Autodesk Inventor part; units mm, degrees
ref_plane "YZ Plane" through (0, 0, 0) normal (1, 0, 0) x (0, 1, 0)
ref_plane "XZ Plane" through (0, 0, 0) normal (0, 1, 0) x (-1, 0, 0)
ref_plane "XY Plane" through (0, 0, 0) normal (0, 0, 1) x (1, 0, 0)
sketch "Sketch1" plane through (0, 0, 0) normal (0, 1, 0) x (-1, 0, 0)
  line L0 (-7.5692, 28.702) -> (7.5692, 28.702) construction
  line L1 (7.5692, 28.702) -> (7.5692, -28.702) construction
  line L2 (7.5692, -28.702) -> (-7.5692, -28.702) construction
  line L3 (-7.5692, -28.702) -> (-7.5692, 28.702) construction
  line L4 (-7.5692, 28.702) -> (7.5692, -28.702) construction
  line L5 (7.5692, 28.702) -> (-7.5692, -28.702) construction
  line L6 (-4.3815, -7.5692) -> (4.3815, -7.5692)
  line L7 (4.3815, -7.5692) -> (4.3815, 7.5692)
  line L8 (4.3815, 7.5692) -> (-4.3815, 7.5692)
  line L9 (-4.3815, 7.5692) -> (-4.3815, -7.5692)
  line L10 (-4.3815, -7.5692) -> (4.3815, 7.5692) construction
  line L11 (4.3815, -7.5692) -> (-4.3815, 7.5692) construction
  line L12 (-7.5692, -28.702) -> (-3.3782, -28.702)
  line L13 (7.5692, -17.78) -> (-3.3782, -28.702)
  line L14 (-7.5692, -28.702) -> (-7.5692, 0)
  line L15 (21.6792, 0) -> (-18.0822, 0) construction
  line L16 (-7.5692, 28.702) -> (-7.5692, 0)
  line L17 (7.5692, 0) -> (7.5692, -17.78)
  line L18 (7.5692, 0) -> (7.5692, 17.78)
  line L19 (-7.5692, 28.702) -> (0, 28.702)
  line L20 (7.5692, 17.78) -> (0, 28.702)
  point P0 (0, 0)
  point P1 (0, -15.8496)
  point P2 (0, 15.8496)
  point P3 (0, 0)
  dimension "d0" = 57.404
  dimension "d1" = 15.1384
  dimension "d2" = 8.763
  dimension "d3" = 15.1384
  dimension "d4" = 10.9474
  dimension "d5" = 10.922
  dimension "d7" = 7.5692
  dimension "d20" = 10.922
  dimension "d21" = 7.5692
  dimension "mounting_hole_distance" = 31.6992
extrude "Extrusion2" add sketch "Sketch1" against normal blind 1.5748
hole "Hole1" at (0, 0, -15.8496) at (0, 0, 15.8496) direction (0, -1, 0) diameter 2.159 depth 8.8646 tip angle 118
equation "\"d20\" = d5"
equation "\"d21\" = d7"
properties part number "orginal_headplate_ben"
Build history of the part. All positions in model axes, mm. A direction names the side the tool comes from. Round coordinates to 2 decimals unless told otherwise and drop trailing zeros. Loops run counter-clockwise (first coordinate to the right, second up) from the corner with the lowest first, then second, coordinate; pieces in that order, holes last. Notation, with made-up numbers: (65.25, 45.5) -> (108.25, 45.5) arc R30 ccw to (108.25, 73.5) -> close; hole circle Ø8 at (81, -2.5). An arc over 180 degrees is marked (long way). Use CSV: the item, a comma, the result in double quotes. Start each with the question number.
Q1. Mould opens along X. For faces 1 (the face through (7.569, -1, 0)), 2 (the face through (5, 0, 0)), 3 (the face through (-0.047, -0.798, -16.928)), 4 (the face through (-7.569, -1, 0)) say: +X half, -X half, draft (parallel to the pull), parting line (faces both ways), or undercut.
Q2. Saw through at C-C on x = -3.5. Give the cut face in (y, z), and give its area (3 significant figures).
Q3. Saw through at A-A on x = 1.75. Give the cut face in (y, z).
Q4. Saw through at B-B on y = -0.9. Give the cut face in (x, z), and give its area (3 significant figures).
Q5. Which spindle directions (+Z, -Z, +X, -X, +Y, -Y) get a long thin tool onto all of the face, cutting with end or side? Do faces 5 (the face through (4.382, -1, 0)), 6 (the face through (-3.84, -0.78, 23.16)). Say none if no direction does.
Q6. Drill centre lines: L1, parallel to X at y = -0.3, z = -6.5; L2, parallel to Z at x = 0, y = -0.55; L3, parallel to X at y = -0.55, z = 15.5. Where is each one in solid material? Low to high.
Solutions:
1,face 1,"+X half"
1,face 2,"draft"
1,face 3,"undercut"
1,face 4,"-X half"
2,outline,"(-1.57, -21.84) -> (0, -21.84) -> (0, -7.57) -> (-1.57, -7.57) -> close; (-1.57, 7.57) -> (0, 7.57) -> (0, 23.65) -> (-1.57, 23.65) -> close"
2,area,"47.8 mm^2"
3,outline,"(-1.57, -27.08) -> (0, -27.08) -> (0, -7.57) -> (-1.57, -7.57) -> close; (-1.57, 7.57) -> (0, 7.57) -> (0, 28.7) -> (-1.57, 28.7) -> close"
4,outline,"(-7.57, -17.78) -> (3.38, -28.7) -> (7.57, -28.7) -> (7.57, 28.7) -> (0, 28.7) -> (-7.57, 17.78) -> close; hole (-4.38, -7.57) -> (4.38, -7.57) -> (4.38, 7.57) -> (-4.38, 7.57) -> close; hole circle Ø2.16 at (0, -15.85); hole circle Ø2.16 at (0, 15.85)"
4,area,"628 mm^2"
5,face 5,"+Y, -Y"
5,face 6,"+Z, -X, +Y, -Y"
6,L1,"x = -7.57 to -4.38, 4.38 to 7.57"
6,L2,"z = -25.33 to -16.93, -14.77 to -7.57, 7.57 to 14.77, 16.93 to 28.7"
6,L3,"x = -7.57 to -1.02, 1.02 to 7.57"
